The figure shows three views and two pictorial views of one solid part (mm, origin at its lowest corner). Answer the questions. A direction names the side the tool comes from. Give positions to 0.01 mm unless a question says otherwise; leave off trailing zeros. Loops run counter-clockwise (first coordinate to the right, second up) from the corner with the lowest first, then second, coordinate; pieces in that order, holes last. Notation, with made-up numbers: (-25, -18.5) - (-18, -18.5) arc R21 ccw to (-18, 9.5) - close; hole circle Ø9 at (12, 39.5). An arc over 180 degrees is marked (long way). Write each question's results on one line, items separated by ' | '.
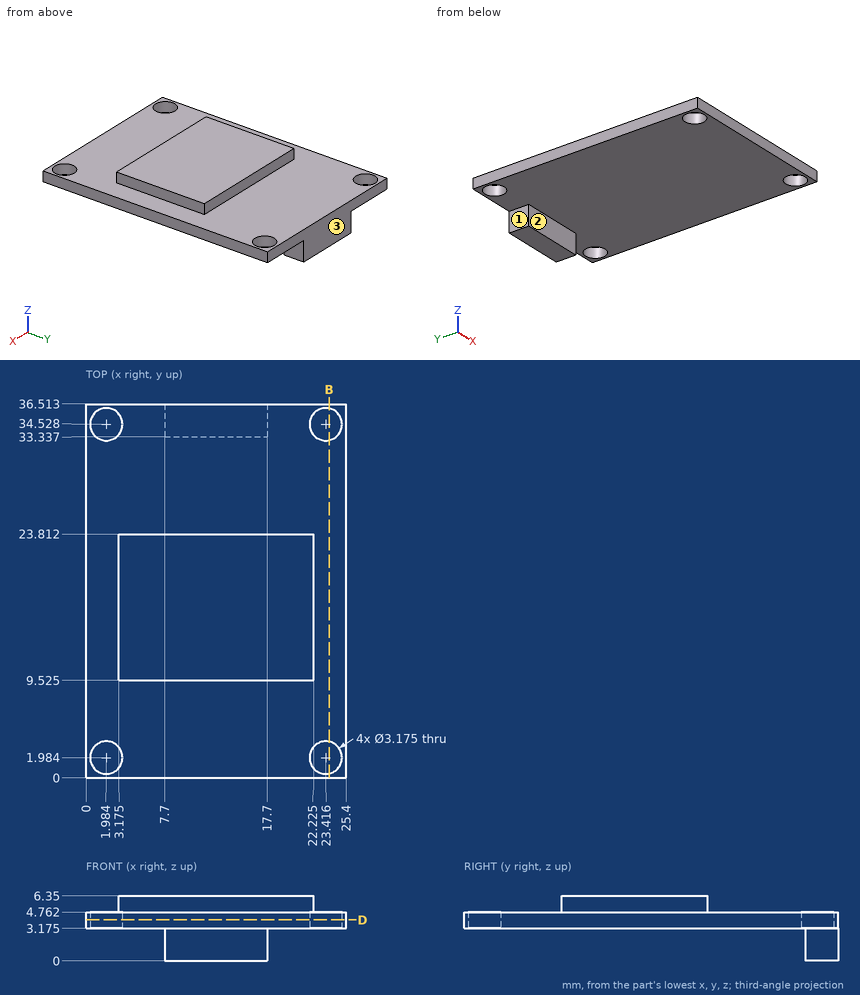
Item 1: A cutting plane is placed at B-B, the plane x = 23.75. Determine the outline of the cut face in (y, z) (1 decimal).
Values found:
outline: (0, 3.2) - (0.4, 3.2) - (0.4, 4.8) - (0, 4.8) - close; (3.5, 3.2) - (33, 3.2) - (33, 4.8) - (3.5, 4.8) - close; (36.1, 3.2) - (36.5, 3.2) - (36.5, 4.8) - (36.1, 4.8) - close
Item 2: Find the intervals of material crossed by line 1 along Y through (x, z) = (2.25, 4.5); line 2 along X through (y, z) = (35.5, 4.25); line 3 along Z through (x, y) = (23.5, 28) (1 decimal), in increasing order. Write a range as [from, to].
Values found:
line 1: y = [0, 0.42], [3.55, 32.96], [36.09, 36.51] | line 2: x = [0, 0.73], [3.24, 22.16], [24.67, 25.4] | line 3: z = [3.2, 4.8]
Item 3: For the marked faces 1, 2 and 3, determine the directions among +Z, -Z, +X, -X, +Y, -Y from which every point of the face is accessible in a straight line to the end or side of a thin tool.
Values found:
face 1: -Z, -X, +Y, -Y | face 2: -Z, +X, -X, -Y | face 3: +Z, -Z, +X, -X, +Y
Item 4: A cutting plane is placed at D-D, the plane z = 4. Determine the outline of the cut face in (x, y) (1 decimal), plus the area to 3 significant figures.
Values found:
outline: (0, 0) - (25.4, 0) - (25.4, 36.5) - (0, 36.5) - close; hole circle Ø3.2 at (2, 2); hole circle Ø3.2 at (2, 34.5); hole circle Ø3.2 at (23.4, 2); hole circle Ø3.2 at (23.4, 34.5) | area: 896 mm²
Item 5: Flat-ended cylindrical pins translate along their axes: P1, Ø5, axis at x = 10.5, y = 29, coming from the +Z side; P2, Ø2.5, axis at x = 23.42, y = 34.53, coming from the +Z side; P3, Ø4, axis at x = 19, y = 20, coming from the -Z side (1 decimal); P4, Ø0.8, axis at x = 13.5, z = 5.5, coming from the -Y side (1 decimal). Find the tip coordinate at first contact, or state that the pin passes through.
Values found:
P1: stops at z = 4.76 | P2: passes through | P3: stops at z = 3.2 | P4: stops at y = 9.5
